Autodesk Inventor part; units mm, degrees
ref_plane "YZ Plane" through (0, 0, 0) normal (1, 0, 0) x (0, 1, 0)
ref_plane "XZ Plane" through (0, 0, 0) normal (0, 1, 0) x (-1, 0, 0)
ref_plane "XY Plane" through (0, 0, 0) normal (0, 0, 1) x (1, 0, 0)
sketch "Эскиз1" plane through (0, 0, 0) normal (0, 1, 0) x (-1, 0, 0)
  line L0 (16.8789, 0) -> (-16.2789, 0)
  arc A0 (16.2789, -0.6) -> (16.8789, 0) centre (16.2789, 0) ccw
  line L1 (16.2789, -0.6) -> (7.2789, -0.6)
  line L2 (7.2789, -0.6) -> (7.2789, -0.85)
  line L3 (7.2789, -0.85) -> (-1.1211, -0.85)
  line L4 (-1.1211, -0.85) -> (-1.1211, 0)
  point P0 (0, 0)
  point P1 (0, 0)
  dimension "pin_small_rad" = 0.6
  dimension "d1" = 18
  dimension "d2" = 9
  dimension "pin_big_dia" = 1.7
revolve "Вращение1" add sketch "Эскиз1" angle 360 about axis through (-16.8789, 0, 0) along (1, 0, 0)
hole "Отверстие1" at (1.1211, 0, 0) direction (-1, 0, 0) diameter 1 depth 2.5 tip angle 118
properties part number "kls_pin" material "Сталь, нержавеющая, полированная"
Geometry check sheet. Reference: the model listing, model coordinates, mm. A direction names the side the tool comes from. Give positions to 0.01 mm unless a question says otherwise; leave off trailing zeros. Order: outer loops, then holes, each group sorted by start corner. A loop starts at its lowest first (then second) coordinate and runs counter-clockwise, first axis right, second up. Notation, with made-up numbers: (18.25, -15) - (63.25, -15) arc R23 cw to (63.25, 23) - close; hole circle Ø6 at (-26, 33.25). An arc over 180 degrees is marked (long way). Use one line per item in the form item = value.
1) Access from +Z, -Z, +X, -X, +Y, -Y to the whole of each face (thin tool, end or side, straight path). Record for faces 1 (the face through (-0.146, 0.488, 0.108)), 2 (the face through (-3.02, -0.83, 0.18)).
Working result:
face_1 = +X
face_2 = +X, -X
2) Sectioned sample at A-A (x = -14.75). Record the boundary of the cut face in (y, z).
Working result:
outline = circle Ø1.2 at (0, 0)
3) Material ranges on probe 1 along Y at (x, z) = (-0.15, 0); probe 2 along X at (y, z) = (0.5, 0.5); probe 3 along X at (y, z) = (-0.15, 0), recorded low to high. Write a range as from..to.
Working result:
probe_1 = -0.85..-0.5, 0.5..0.85
probe_2 = -7.28..1.12
probe_3 = -16.86..-1.59
4) Draft check along Z on faces 3 (the face through (-11.716, 0.506, -0.323)), 4 (the face through (-1.63, -0.08, 0.02)). Enter one of: released by +Z, released by -Z, zero draft, split by the parting line, or undercut.
Working result:
face_3 = split by the parting line
face_4 = undercut
5) Sectioned sample at B-B (x = -3). Record the boundary of the cut face in (y, z), and give its area (3 significant figures).
Working result:
outline = circle Ø1.7 at (0, 0)
area = 2.27 mm^2
